Input: part model. Units: mm. Frame: model coordinates. Face numbers are marked on the shaded views. A direction names the side the tool comes from. Give positions to 0.01 mm unless a question says otherwise; leave off trailing zeros. Write each loop counter-clockwise with the first axis right and the second up, starting at its lowest first coordinate (ties: lowest second). Pieces come first, ordered by that corner, then holes. Notation, with made-up numbers: (57.5, 79) -> (94.5, 79) arc R16 cw to (94.5, 93) -> close; hole circle Ø10 at (8, 18). An arc over 180 degrees is marked (long way). Answer as a JSON object with one key per item and string values. Group by question number.
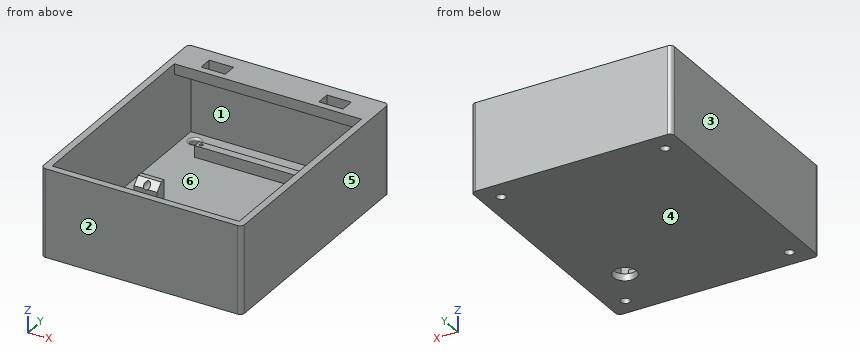
Autodesk Inventor part; units mm, degrees
ref_plane "YZ Plane" through (0, 0, 0) normal (1, 0, 0) x (0, 1, 0)
ref_plane "XZ Plane" through (0, 0, 0) normal (0, 1, 0) x (-1, 0, 0)
ref_plane "XY Plane" through (0, 0, 0) normal (0, 0, 1) x (1, 0, 0)
sketch "Sketch1" plane through (0, 0, 0) normal (0, 0, 1) x (1, 0, 0)
  line L0 (25.0097, 21.6893) -> (25.0097, -75.3107)
  line L1 (-44.9903, 13.4393) -> (14.5097, 13.4393)
  line L2 (14.5097, 13.4393) -> (14.5097, -66.5607)
  line L3 (14.5097, -66.5607) -> (-44.9903, -66.5607)
  line L4 (-44.9903, -66.5607) -> (-44.9903, 13.4393)
  circle A0 centre (12.7597, 11.6893) radius 0.75
  circle A1 centre (-43.2403, 11.6893) radius 0.75
  circle A2 centre (-43.2403, -64.8107) radius 0.75
  circle A3 centre (12.7597, -64.8107) radius 0.75
  line L5 (-44.9903, 13.4393) -> (14.5097, 13.4393)
  line L6 (14.5097, 13.4393) -> (14.5097, 9.9393)
  line L7 (14.5097, 9.9393) -> (-44.9903, 9.9393)
  line L8 (-44.9903, 9.9393) -> (-44.9903, 13.4393)
  line L9 (14.5097, -66.5607) -> (-44.9903, -66.5607)
  line L10 (-44.9903, -66.5607) -> (-44.9903, -63.0607)
  line L11 (-44.9903, -63.0607) -> (14.5097, -63.0607)
  line L12 (14.5097, -63.0607) -> (14.5097, -66.5607)
  circle A4 centre (-50.9903, 20.1893) radius 2
  circle A5 centre (20.0097, 20.1893) radius 2
  circle A6 centre (20.0097, -70.3107) radius 2
  circle A7 centre (-50.9903, -70.3107) radius 2
  line L13 (-55.9903, 25.6893) -> (25.0097, 25.6893)
  line L14 (25.0097, 25.6893) -> (25.0097, -75.3107)
  line L15 (25.0097, -75.3107) -> (-55.9903, -75.3107)
  line L16 (-55.9903, -75.3107) -> (-55.9903, 25.6893)
  line L17 (-55.9903, 10.6893) -> (-55.9903, 17.6893)
  line L18 (25.0097, 10.1893) -> (25.0097, 17.1893)
  line L19 (-58.9903, 28.6893) -> (28.0097, 28.6893)
  line L20 (28.0097, 28.6893) -> (28.0097, -78.3107)
  line L21 (28.0097, -78.3107) -> (-58.9903, -78.3107)
  line L22 (-58.9903, -78.3107) -> (-58.9903, 28.6893)
  point P0 (0, 0)
  point P1 (-14.9903, -76.5607)
  point P2 (-44.9903, 9.9393)
  point P3 (14.5097, 9.9393)
  point P4 (14.5097, -63.0607)
  point P5 (-44.9903, -63.0607)
  dimension "d4" = 10
  dimension "d5" = 10.5
  dimension "d6" = 1.5
  dimension "d7" = 1.5
  dimension "d8" = 1.5
  dimension "d9" = 1.5
  dimension "d11" = 1.75
  dimension "d12" = 1.75
  dimension "d13" = 1.75
  dimension "d14" = 1.75
  dimension "d15" = 1.75
  dimension "d16" = 1.75
  dimension "d17" = 1.75
  dimension "d18" = 1.75
  dimension "d20" = 0
  dimension "d21" = 0
  dimension "d22" = 3.5
  dimension "d24" = 0
  dimension "d25" = 3.5
  dimension "d26" = 0
  dimension "d39" = 4
  dimension "d42" = 4
  dimension "d43" = 4
  dimension "d44" = 4
  dimension "d46" = 5
  dimension "d47" = 5
  dimension "d70" = 81
  dimension "d71" = 101
  dimension "d75" = 5.5
  dimension "d111" = 87
  dimension "d112" = 107
  dimension "d113" = 3
  dimension "d114" = 3
  dimension "d115" = 5
  dimension "d116" = 5
  dimension "d117" = 5
  dimension "d125" = 3
  dimension "d126" = 5
  dimension "d127" = 5.5
  dimension "d128" = 11
  dimension "d129" = 3
extrude "Extrusion5" add sketch "Sketch1" against normal blind 3 contours L0 L15 L16 L13 L14 | L1 L2 L7 L4 | L7 L2 L11 L4 | L11 L2 L3 L4 | A0 | A1 | A2 | A3 | A4 | A5 | A6 | A7 | L19 L20 L21 L22
extrude "Extrusion7" add sketch "Sketch1" along normal blind 5 contours L1 L2 L7 L4 | L11 L2 L3 L4
extrude "Extrusion11" cut sketch "Sketch1" against normal blind 200 contours A4 | A5 | A6 | A7
fillet "Fillet3" radius 1 4 edges at (-52.9903, 20.1893, 0) (18.0097, 20.1893, 0) (18.0097, -70.3107, 0) (-52.9903, -70.3107, 0)
extrude "Extrusion17" add sketch "Sketch1" along normal blind 35 contours L19 L20 L21 L22
sketch "Sketch9" plane through (-55.9903, -75.3107, 0) normal (1, 0, 0) x (0, 0, -1)
  line L0 (-35, 0) -> (-35, 101)
  line L1 (-35, 101) -> (-30.5, 101)
  line L2 (-30.5, 101) -> (-30.5, 89)
  line L3 (-30.5, 89) -> (-35, 89)
  line L4 (-35, 89) -> (-35, 101)
  point P0 (0, 75.3107)
  point P1 (-35, 89)
  dimension "d120" = 4.5
  dimension "d121" = 12
extrude "Extrusion18" add sketch "Sketch9" along normal blind 81
fillet "Fillet4" radius 2 4 edges at (-58.9903, 28.6893, 16) (28.0097, 28.6893, 16) (28.0097, -78.3107, 16) (-58.9903, -78.3107, 16)
sketch "Sketch11" plane through (-55.9903, 13.6893, 30.5) normal (0, 0, -1) x (-1, 0, 0)
  line L0 (-71.25, 9) -> (-60.75, 9)
  line L1 (-60.75, 9) -> (-60.75, 3)
  line L2 (-60.75, 3) -> (-71.25, 3)
  line L3 (-71.25, 3) -> (-71.25, 9)
  line L4 (-81, 0) -> (-81, 12)
  line L5 (-81, 12) -> (0, 12)
  line L6 (0, 12) -> (0, 0)
  line L7 (-20.25, 9) -> (-9.75, 9)
  line L8 (-9.75, 9) -> (-9.75, 3)
  line L9 (-9.75, 3) -> (-20.25, 3)
  line L10 (-20.25, 3) -> (-20.25, 9)
  point P0 (-55.9903, -13.6893)
  dimension "d130" = 6
  dimension "d131" = 9.75
  dimension "d132" = 10.5
  dimension "d133" = 3
  dimension "d137" = 9.75
  dimension "d138" = 10.5
  dimension "d139" = 6
  dimension "d140" = 3
extrude "Extrusion19" cut sketch "Sketch11" against normal blind 5
sketch "Sketch12" plane through (-55.9903, -75.3107, 0) normal (0, 1, 0) x (1, 0, 0)
  line L0 (35.5, -35) -> (45.5, -35)
  line L1 (45.5, -35) -> (45.5, -30)
  line L2 (45.5, -30) -> (35.5, -30)
  line L3 (35.5, -30) -> (35.5, -35)
  line L4 (0, 0) -> (0, -35)
  line L5 (81, -35) -> (0, -35)
  line L6 (81, 0) -> (81, -35)
  point P0 (55.9903, 0)
  dimension "d143" = 35.5
  dimension "d144" = 0
  dimension "d146" = 5
  dimension "d147" = 10
  dimension "d148" = 35.5
extrude "Extrusion20" add sketch "Sketch12" along normal blind 5
sketch "Sketch13" plane through (0, 0, 35) normal (0, 0, 1) x (1, 0, 0)
  line L0 (-20.4903, -70.3107) -> (-10.4903, -70.3107)
  line L1 (-20.4903, -75.3107) -> (-10.4903, -75.3107)
  line L2 (-20.4903, -70.3107) -> (-10.4903, -70.3107)
  line L3 (-10.4903, -70.3107) -> (-10.4903, -75.3107)
  line L4 (-10.4903, -75.3107) -> (-20.4903, -75.3107)
  line L5 (-20.4903, -75.3107) -> (-20.4903, -70.3107)
  point P0 (0, 0)
extrude "Extrusion21" add sketch "Sketch13" along normal blind 5
chamfer "Chamfer3" distance 3 angle 45 1 edges at (-15.4903, -75.3107, 40)
sketch "Sketch14" plane through (-55.9903, -70.3107, 0) normal (0, 1, 0) x (1, 0, 0)
  circle A0 centre (40.5, -38) radius 1.375
  line L0 (45.5, -30) -> (45.5, -40)
  line L1 (35.5, -30) -> (35.5, -40)
  line L2 (45.5, -30) -> (35.5, -30)
  line L3 (45.5, -40) -> (35.5, -40)
  point P0 (55.9903, 0)
  point P1 (40.5, -30)
  point P2 (40.5, -40)
  dimension "d156" = 2.75
  dimension "d157" = 5
  dimension "d158" = 5
  dimension "d159" = 8
  dimension "d160" = 2
extrude "Extrusion22" cut sketch "Sketch14" against normal blind 5 contours A0
sketch "Sketch15" plane through (0, 0, 0) normal (0, 0, 1) x (1, 0, 0)
  circle A0 centre (10.0097, -53.0607) radius 5
  line L0 (25.0097, 13.6893) -> (25.0097, -75.3107)
  line L1 (14.5097, -63.0607) -> (-44.9903, -63.0607)
  point P0 (0, 0)
  dimension "d163" = 15
  dimension "d164" = 10
  dimension "d165" = 10
extrude "Extrusion23" cut sketch "Sketch15" against normal blind 5
properties part number "Backboard deel 1"
1. Section D-D (x = -5.5). Return the cut outline in (y, z), plus the area to 3 significant figures.
2. Mould query, pull axis X, two halves, no side actions, for the marked faces 3, 4, 5 and 6. Classes: pulls with the +X half, pulls with the -X half, needs draft (parallel to the pull), parting line crosses it, or undercut.
3. Reachability of the marked faces 1 and 2 from +Z, -Z, +X, -X, +Y, -Y: full face, straight path, thin tool, end or side. Return the list, or none.
4. Line query: line 1 (Y direction, x = -36.5, z = 32.5); line 2 (Y direction, x = 3, z = 28); line 3 (X direction, y = -21, z = 18.5). Output: solid intervals per line, ascending.
5. Contact query for flat-ended pins moving along their axis: pin 1 Ø2 at (x, y) = (-17.5, -56.5) entering from +Z; pin 2 Ø3 at (x, y) = (-50.99, 20.19) entering from -Z; pin 3 Ø2.5 at (x, y) = (12.76, 11.69) entering from +Z; pin 4 Ø2.5 at (x, y) = (20.01, -70.31) entering from -Z (3 decimals). Output: stop coordinate, or through.
6. Section B-B (z = 15). Return the cut outline in (x, y).
7. Section C-C (y = 7.5). Return the cut outline in (x, z), plus the area to 3 significant figures.
8. Section A-A (x = -38.5). Return the cut outline in (y, z), plus the area to 3 significant figures.
Working result:
{
 "1": {"outline": "(-78.31, -3) -> (28.69, -3) -> (28.69, 35) -> (13.69, 35) -> (13.69, 30.5) -> (25.69, 30.5) -> (25.69, 0) -> (13.44, 0) -> (13.44, 5) -> (9.94, 5) -> (9.94, 0) -> (-63.06, 0) -> (-63.06, 5) -> (-66.56, 5) -> (-66.56, 0) -> (-75.31, 0) -> (-75.31, 35) -> (-78.31, 35) -> close", "area": "620 mm^2"},
 "2": {"face 3": "pulls with the -X half", "face 4": "needs draft", "face 5": "pulls with the +X half", "face 6": "undercut"},
 "3": {"face 1": "none", "face 2": "+Z, -Z, +X, -X, -Y"},
 "4": {"line 1": "y = -78.31 to -75.31, 13.69 to 16.69, 22.69 to 28.69", "line 2": "y = -78.31 to -75.31, 25.69 to 28.69", "line 3": "x = -58.99 to -55.99, 25.01 to 28.01"},
 "5": {"pin 1": "stops at z = 0", "pin 2": "stops at z = 30.5", "pin 3": "stops at z = 5", "pin 4": "passes through"},
 "6": {"outline": "(-58.99, -76.31) arc R2 ccw to (-56.99, -78.31) -> (26.01, -78.31) arc R2 ccw to (28.01, -76.31) -> (28.01, 26.69) arc R2 ccw to (26.01, 28.69) -> (-56.99, 28.69) arc R2 ccw to (-58.99, 26.69) -> close; hole (-55.99, -75.31) -> (25.01, -75.31) -> (25.01, 25.69) -> (-55.99, 25.69) -> close"},
 "7": {"outline": "(-58.99, -3) -> (28.01, -3) -> (28.01, 35) -> (25.01, 35) -> (25.01, 0) -> (-55.99, 0) -> (-55.99, 35) -> (-58.99, 35) -> close", "area": "471 mm^2"},
 "8": {"outline": "(-78.31, -3) -> (28.69, -3) -> (28.69, 35) -> (22.69, 35) -> (22.69, 30.5) -> (25.69, 30.5) -> (25.69, 0) -> (13.44, 0) -> (13.44, 5) -> (9.94, 5) -> (9.94, 0) -> (-63.06, 0) -> (-63.06, 5) -> (-66.56, 5) -> (-66.56, 0) -> (-75.31, 0) -> (-75.31, 35) -> (-78.31, 35) -> close; (13.69, 30.5) -> (16.69, 30.5) -> (16.69, 35) -> (13.69, 35) -> close", "area": "593 mm^2"}
}
